Verification items for this drawing (mm, ordinates from the low corner). Give positions to 0.01 mm unless a question says otherwise; leave off trailing zeros. Use one line per item in the form item = value. Start each with the question number.
(1) Release check for a two-part mould opening along X. For the marked faces 1, 2 and 3 record: pulls with the +X half, pulls with the -X half, needs draft (parallel to the pull), parting line crosses it, or undercut.
(2) Scan lines: L1, parallel to X at y = 9.75, z = 58.5; L2, parallel to X at y = 10.75, z = 6 (1 decimal); L3, parallel to Z at x = 21, y = 22 (1 decimal). Record each from-to range of solid material in increasing order.
(3) Section check A-A, the plane z = 85. State how many separate pieces and enclosed holes the cut face has, plus the area to 3 significant figures.
(4) Depth check by flat-ended pin: pin 1 Ø1 at (y, z) = (19, 45) entering from -X. Enter the tip coordinate at first touch or a pass-through.
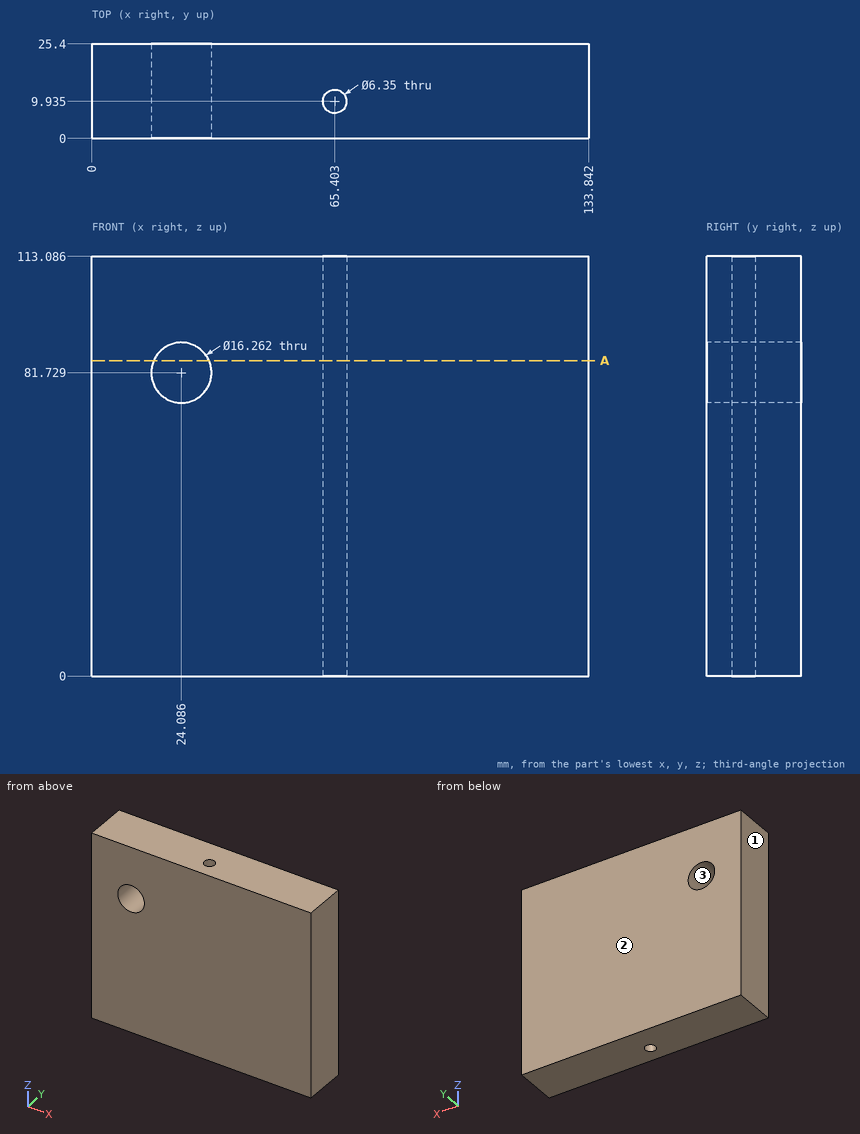
Completed:
q1.face_1 = pulls with the -X half
q1.face_2 = needs draft
q1.face_3 = undercut
q2.L1 = 0 to 62.23, 68.57 to 133.84
q2.L2 = 0 to 62.3, 68.5 to 133.8
q2.L3 = 0 to 74.2, 89.3 to 113.1
q3.separate_pieces = 2
q3.enclosed_holes = 1
q3.area = 2,990 mm²
q4.pin_1 = 0
